Check sheet for the modelled part. Datum: model origin and axes. Units: mm. Round coordinates to 2 decimals unless told otherwise and drop trailing zeros. Order: outer loops, then holes, each group sorted by start corner. A loop starts at its lowest first (then second) coordinate and runs counter-clockwise, first axis right, second up. Notation, with made-up numbers: (44.5, 14) -> (52.5, 14) arc R31 ccw to (52.5, 51) -> close; hole circle Ø11 at (68.5, 23.5). An arc over 180 degrees is marked (long way). Answer in a Markdown table with one row per item.
from build123d import *

# Parameters (mm, degrees)
BOSS_EXTRUDE1_DEPTH = 237


with BuildPart() as part:
    # Sketch1 → Boss-Extrude1 (new body)
    with BuildSketch(Plane(origin=(0, 0, 0), x_dir=(0, 0, -1), z_dir=(1, 0, 0))):
        with BuildLine():
            Line((2.397915762, 5.5), (-2.397915762, 5.5))
            ThreePointArc((-2.397915762, 5.5), (-3, 5.196152423), (-3.56418184, 4.826655966))
            Line((-3.56418184, 4.826655966), (-5.962097602, 0.673344034))
            ThreePointArc((-5.962097602, 0.673344034), (-6, 0), (-5.962097602, -0.673344034))
            Line((-5.962097602, -0.673344034), (-3.56418184, -4.826655966))
            ThreePointArc((-3.56418184, -4.826655966), (-3, -5.196152423), (-2.397915762, -5.5))
            Line((-2.397915762, -5.5), (2.397915762, -5.5))
            ThreePointArc((2.397915762, -5.5), (3, -5.196152423), (3.56418184, -4.826655966))
            Line((3.56418184, -4.826655966), (5.962097602, -0.673344034))
            ThreePointArc((5.962097602, -0.673344034), (6, 0), (5.962097602, 0.673344034))
            Line((5.962097602, 0.673344034), (3.56418184, 4.826655966))
            ThreePointArc((3.56418184, 4.826655966), (3, 5.196152423), (2.397915762, 5.5))
        make_face()
    extrude(amount=BOSS_EXTRUDE1_DEPTH)

    # Sketch3 → Cut-Revolve6 (revolve, cut)
    with BuildSketch(Plane(origin=(0, 0, 0), x_dir=(1, 0, 0), z_dir=(0, 1, 0))):
        Polygon((236.5, -6), (237, -6), (237, -5.5), align=None)
    revolve(axis=Axis((0, 0, 0), (1, 0, 0)), mode=Mode.SUBTRACT)

    # Mirror1: part across plane


with BuildPart() as part_1:
    add(part.part)
    add(part.part.mirror(Plane(origin=(0, 0, 0), x_dir=(0, 0, 1), z_dir=(1, 0, 0))))


solid = part_1.part
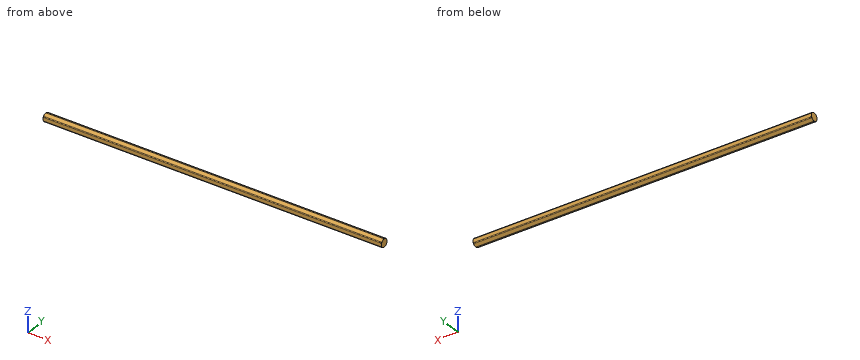
Item 1: Scan lines: line 1 (Z direction, x = -169.5, y = -2.75); line 2 (Z direction, x = 56, y = 0.5); line 3 (Y direction, x = 209, z = -2.5). Record each from-to range of solid material in increasing order. Write a range as [from, to].
Result sheet:
| item | result |
|---|---|
| line 1 | z = [-4.76, 4.76] |
| line 2 | z = [-5.98, 5.98] |
| line 3 | y = [-5.45, 5.45] |
Item 2: Depth check by flat-ended pin: P1, Ø4, axis at x = 1, y = -3, coming from the +Z side; P2, Ø4, axis at x = 49, y = 3, coming from the -Z side; P3, Ø1, axis at x = 79, z = 3, coming from the +Y side. Enter the tip coordinate at first touch or a pass-through.
Result sheet:
| item | result |
|---|---|
| P1 | stops at z = 5.77 |
| P2 | stops at z = -5.77 |
| P3 | stops at y = 5.45 |
Item 3: Cross-section at A-A (x = -199). Record the boundary of the cut face in (y, z), and give its area (3 significant figures).
Result sheet:
| item | result |
|---|---|
| outline | (-5.5, -2.4) arc R6 ccw to (-4.83, -3.56) -> (-0.67, -5.96) arc R6 ccw to (0.67, -5.96) -> (4.83, -3.56) arc R6 ccw to (5.5, -2.4) -> (5.5, 2.4) arc R6 ccw to (4.83, 3.56) -> (0.67, 5.96) arc R6 ccw to (-0.67, 5.96) -> (-4.83, 3.56) arc R6 ccw to (-5.5, 2.4) -> close |
| area | 103 mm^2 |
